```python
from build123d import *

# Parameters (mm, degrees)
BASEPLATESKETCH_W   = 50
BASEPLATESKETCH_H   = 50
BOSS_EXTRUDE1_DEPTH = 10
SKETCH2_R           = 5
BOSS_EXTRUDE3_DEPTH = 100
LPATTERN1_COUNT     = 2
LPATTERN1_PITCH     = 12.5
LPATTERN1_COL_COUNT = 2
LPATTERN1_COL_PITCH = 12.5
SKETCH7_W           = 50
SKETCH7_H           = 51
BOSS_EXTRUDE4_DEPTH = 10


with BuildPart() as part:
    # baseplatesketch → Boss-Extrude1 (new body)
    with BuildSketch(Plane(origin=(0, 0, 0), x_dir=(0, 0, -1), z_dir=(1, 0, 0))):
        Rectangle(BASEPLATESKETCH_W, BASEPLATESKETCH_H)
    extrude(amount=BOSS_EXTRUDE1_DEPTH)

    # Sketch2 → Boss-Extrude3 (add)
    with BuildSketch(Plane(origin=(10, 0, 0), x_dir=(0, 0, -1), z_dir=(1, 0, 0))):
        Circle(SKETCH2_R)
    boss_extrude3 = extrude(amount=BOSS_EXTRUDE3_DEPTH)

    # LPattern1: Boss-Extrude3 ×2
    with Locations(*[(0, 0, -i * LPATTERN1_PITCH) for i in range(1, LPATTERN1_COUNT)]):
        add(boss_extrude3)

    # LPattern1 col: Boss-Extrude3 ×2
    with Locations(*[(0, 0, i * LPATTERN1_COL_PITCH) for i in range(1, LPATTERN1_COL_COUNT)]):
        add(boss_extrude3)

    # Sketch7 → Boss-Extrude4 (add)
    with BuildSketch(Plane(origin=(110, 0, 0), x_dir=(0, 0, -1), z_dir=(1, 0, 0))):
        with Locations((0, -0.5)):
            Rectangle(SKETCH7_W, SKETCH7_H)
    extrude(amount=BOSS_EXTRUDE4_DEPTH)

    # Mirror8: part across plane


with BuildPart() as part_1:
    add(part.part)
    add(part.part.mirror(Plane(origin=(0, -26, 0), x_dir=(0, 0, 1), z_dir=(0, -1, 0))))


solid = part_1.part
```
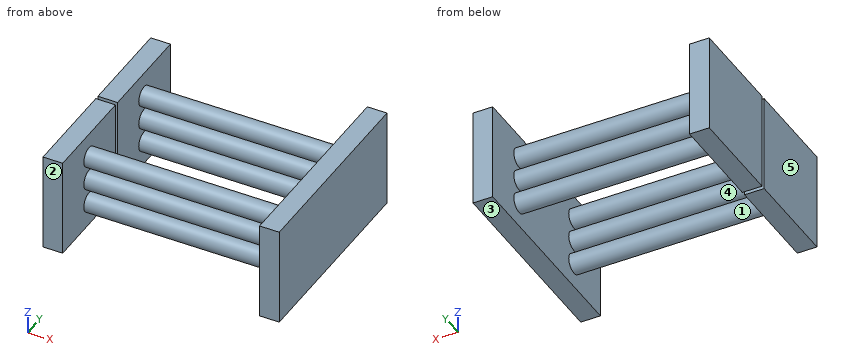
Can you work these out from the model? Positions are in its coordinate system, mm. Face numbers are marked on the shaded views. A direction names the side the tool comes from. Coordinates: 2 decimals unless noted, no trailing zeros. Loops run counter-clockwise (first coordinate to the right, second up) from the corner with the lowest first, then second, coordinate; pieces in that order, holes last. Notation, with made-up numbers: M 81.25,67 L 111.25,67 A12 ccw 111.25,76 Z; hole C 65,-35.75 d11. An arc over 180 degrees is marked long. Put each result on its own line as item: value. Start each with the question number.
(1) Imagine slicing it at D-D on y = 0. List the corners of the cut face in (x, z) for me, and give its area (3 significant figures).
(2) Imagine slicing it at C-C on x = 83.5. List the corners of the cut face in (y, z) for me.
(3) Imagine slicing it at B-B on y = -14.5. List the corners of the cut face in (x, z) for me.
(4) Imagine slicing it at A-A on z = 22.5. List the corners of the cut face in (x, y) for me.
(5) Will these pins go through, and if not, where does the flat tip stop? pin 1 Ø3 at (x, z) = (65, 11.5) entering from -Y; pin 2 Ø8 at (x, y) = (66.5, -58) entering from +Z; pin 3 Ø1 at (x, y) = (47, -3) entering from +Z.
(6) Which directions (+Z, -Z, +X, -X, +Y, -Y) give clear straight access to the entire face, cutting with the end or side of a thin tool? Please do the marked faces 4 and 5.
(7) I need wall thicknesses on probe 1 along X at (y, z) = (-30.5, 3); probe 2 along Y at (x, z) = (105.5, 0.5); probe 3 along Z at (x, y) = (77.5, 0.5). Which ranges of each line are inside material? Lowest first, please.
(8) We'd pull the mould along Z, two halves only. Please class the marked faces 1, 2 and 3: +Z half, -Z half, draft (parallel to the pull), parting line (faces both ways), or undercut.
Worked answers:
1. outline: M 0,-25 L 10,-25 L 10,-17.5 L 110,-17.5 L 110,-25 L 120,-25 L 120,25 L 110,25 L 110,17.5 L 10,17.5 L 10,25 L 0,25 Z; hole M 10,-7.5 L 110,-7.5 L 110,-5 L 10,-5 Z; hole M 10,5 L 110,5 L 110,7.5 L 10,7.5 Z
1. area: 4,000 mm2
2. outline: C -52,-12.5 d10; C -52,0 d10; C -52,12.5 d10; C 0,-12.5 d10; C 0,0 d10; C 0,12.5 d10
3. outline: M 0,-25 L 10,-25 L 10,25 L 0,25 Z; M 110,-25 L 120,-25 L 120,25 L 110,25 Z
4. outline: M 0,-77 L 10,-77 L 10,-27 L 0,-27 Z; M 0,-25 L 10,-25 L 10,25 L 0,25 Z; M 110,-77 L 120,-77 L 120,25 L 110,25 Z
5. pin 1: stops at y = -57
5. pin 2: stops at z = 17.08
5. pin 3: stops at z = 16.83
6. face 4: none
6. face 5: +Z, -Z, -X, +Y, -Y
7. probe 1: x = 0 to 10, 110 to 120
7. probe 2: y = -56.97 to -47.03, -4.97 to 4.97
7. probe 3: z = -17.47 to -7.53, -4.97 to 4.97, 7.53 to 17.47
8. face 1: undercut
8. face 2: draft
8. face 3: -Z half
